from build123d import *

# Parameters (mm, degrees)
SKETCH1_W           = 155
SKETCH1_H           = 84
BOSS_EXTRUDE1_DEPTH = 10
FILLET1_R           = 10
SHELL1_T            = -2
SKETCH2_W           = 5
SKETCH2_H           = 10
CUT_EXTRUDE1_DEPTH  = 89.511298714
FILLET2_R           = 1
FILLET3_R           = 0.25
FILLET4_R           = 1


with BuildPart() as part:
    # Sketch1 → Boss-Extrude1 (new body)
    with BuildSketch(Plane(origin=(0, 0, 0), x_dir=(1, 0, 0), z_dir=(0, 1, 0))):
        Rectangle(SKETCH1_W, SKETCH1_H)
    extrude(amount=BOSS_EXTRUDE1_DEPTH)

    # Fillet1
    fillet1_edges = [part.edges().sort_by_distance(p)[0] for p in [
        (77.5, 5, 42),
        (-77.5, 5, 42),
        (-77.5, 5, -42),
        (77.5, 5, -42),
    ]]
    fillet(fillet1_edges, radius=FILLET1_R)

    # Shell1
    shell1_openings = [part.faces().sort_by_distance(p)[0] for p in [
        (0, 10, 0),
    ]]
    offset(amount=SHELL1_T, openings=shell1_openings, kind=Kind.INTERSECTION)

    # Sketch2 → Cut-Extrude1 (cut, through all)
    with BuildSketch(Plane(origin=(0, 2, 0), x_dir=(1, 0, 0), z_dir=(0, 1, 0))):
        with Locations((-63, 30)):
            Rectangle(SKETCH2_W, SKETCH2_H)
    extrude(amount=-CUT_EXTRUDE1_DEPTH, mode=Mode.SUBTRACT)

    # Fillet2
    fillet2_edges = [part.edges().sort_by_distance(p)[0] for p in [
        (-60.5, 1, -35),
        (-60.5, 1, -25),
        (-65.5, 1, -25),
        (-65.5, 1, -35),
    ]]
    fillet(fillet2_edges, radius=FILLET2_R)

    # Fillet3
    fillet3_edges = [part.edges().sort_by_distance(p)[0] for p in [
        (-60.5, 2, -30),
        (-60.5, 0, -30),
        (-63, 2, -25),
        (-63, 0, -25),
        (-65.5, 2, -30),
        (-65.5, 0, -30),
        (-63, 2, -35),
        (-63, 0, -35),
        (-60.792893219, 2, -25.292893219),
        (-60.792893219, 0, -25.292893219),
        (-65.207106781, 2, -25.292893219),
        (-65.207106781, 0, -25.292893219),
        (-65.207106781, 2, -34.707106781),
        (-65.207106781, 0, -34.707106781),
        (-60.792893219, 2, -34.707106781),
        (-60.792893219, 0, -34.707106781),
    ]]
    fillet(fillet3_edges, radius=FILLET3_R)

    # Fillet4
    fillet4_edges = [part.edges().sort_by_distance(p)[0] for p in [
        (0, 10, 42),
        (-77.5, 10, 0),
        (77.5, 10, 0),
        (0, 10, -42),
        (74.571067812, 10, 39.071067812),
        (74.571067812, 10, -39.071067812),
        (-74.571067812, 10, -39.071067812),
        (-74.571067812, 10, 39.071067812),
        (-75.5, 10, 0),
        (0, 10, 40),
        (75.5, 10, 0),
        (0, 10, -40),
    ]]
    fillet(fillet4_edges, radius=FILLET4_R - 0.0001)  # a hair under: the kernel refuses the full size


solid = part.part
Check sheet for the modelled part. Datum: model origin and axes. Units: mm. A direction names the side the tool comes from. Give positions to 0.01 mm unless a question says otherwise; leave off trailing zeros. Order: outer loops, then holes, each group sorted by start corner. A loop starts at its lowest first (then second) coordinate and runs counter-clockwise, first axis right, second up. Notation, with made-up numbers: (27, -2.75) - (42, -2.75) arc R5 ccw to (42, 1.25) - close; hole circle Ø8 at (27, 68.25). An arc over 180 degrees is marked (long way). Answer as CSV lines item,"result".
1. Tool access check on faces 5 (the face through (-1, 5, -40)), 6 (the face through (74.49, 4.56, 39.15)). Record the directions out of +Z, -Z, +X, -X, +Y, -Y that give a thin tool (end or side, any length) a straight path to the whole face; none if there is none.
Result sheet:
face 5,"+Y"
face 6,"+Z, +X, +Y, -Y"
2. Section check B-B (y = 6.25). Record the boundary of the cut face in (x, z).
Result sheet:
outline,"(-77.5, -32) arc R10 ccw to (-67.5, -42) - (67.5, -42) arc R10 ccw to (77.5, -32) - (77.5, 32) arc R10 ccw to (67.5, 42) - (-67.5, 42) arc R10 ccw to (-77.5, 32) - close; hole (-75.5, -32) arc R8 ccw to (-67.5, -40) - (67.5, -40) arc R8 ccw to (75.5, -32) - (75.5, 32) arc R8 ccw to (67.5, 40) - (-67.5, 40) arc R8 ccw to (-75.5, 32) - close"
3. Go/stop test with a flat-tipped pin: P1, Ø1, axis at x = 4, z = 15, coming from the +Y side. Record where the tip stops, or that it passes through.
Result sheet:
P1,"y = 2"
4. Mould release check, pull along Z, two halves, no side actions. Record for faces 1 (the face through (-73.219, 5.549, 37.594)), 2 (the face through (74.65, 4.56, -38.99)), 3 (the face through (-77.5, 4, 0)), 4 (the face through (73.094, 5.549, 37.719)): released by +Z, released by -Z, zero draft, split by the parting line, or undercut.
Result sheet:
face 1,"undercut"
face 2,"released by -Z"
face 3,"zero draft"
face 4,"undercut"
5. Scan lines: probe 1 along X at (y, z) = (7, -22); probe 2 along Z at (x, y) = (6.5, 7.75); probe 3 along Y at (x, z) = (22, -29). Record each from-to range of solid material in increasing order. Write a range as from..to.
Result sheet:
probe 1,"-77.5..-75.5, 75.5..77.5"
probe 2,"-42..-40, 40..42"
probe 3,"0..2"
